Part model, mm, in its own coordinate system. Face numbers are marked on the shaded views. A direction names the side the tool comes from. Coordinates: 2 decimals unless noted, no trailing zeros. Write each loop counter-clockwise with the first axis right and the second up, starting at its lowest first coordinate (ties: lowest second). Pieces come first, ordered by that corner, then holes. Notation, with made-up numbers: M -12,17 L 41,17 A14 ccw 41,32 Z; hole C 11,3.5 d8. An arc over 180 degrees is marked long. Use a Markdown table: item, result. Add a question column.
Q1. Mould opens along X. For the marked faces 5, 6 and 7 say: released by +X, released by -X, zero draft, split by the parting line, or undercut.
Q2. Slice it at D-D on y = 100. Write the cut outline in (x, z).
Q3. Pin check, flat tips, straight feed: pin 1 Ø8 at (x, z) = (170, 58) entering from +Y; pin 2 Ø6 at (x, z) = (7.5, 183) entering from +Y. Stop position of each tip, or through.
Q4. Slice it at B-B on z = 300. Write the cut outline in (x, y), then the cut area to 3 significant figures.
Q5. Tool access for the marked faces 1, 2, 3 and 4: list every direction of +Z, -Z, +X, -X, +Y, -Y with a clear straight run to the whole face (end or side of a thin tool).
Q6. Slice it at C-C on x = 202.5. Write the cut outline in (y, z), then the cut area to 3 significant figures.
Q7. Slice it at A-A on y = 179. Write the cut outline in (x, z).
Q8. Wall check: L1, parallel to X at y = 167.5, z = 113; L2, parallel to Z at x = -142, y = 162.5; L3, parallel to X at y = 118.5, z = 130. Give the ranges that are in metal, low to high. Write a range as from..to.
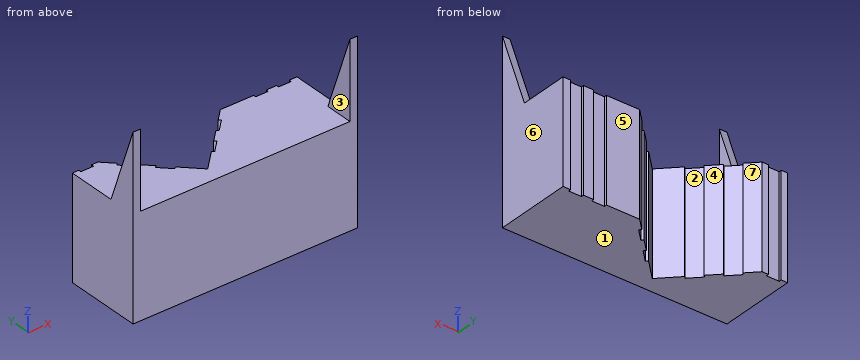
Autodesk Inventor part; units mm, degrees
ref_plane "YZ Plane" through (0, 0, 0) normal (1, 0, 0) x (0, 1, 0)
ref_plane "XZ Plane" through (0, 0, 0) normal (0, 1, 0) x (-1, 0, 0)
ref_plane "XY Plane" through (0, 0, 0) normal (0, 0, 1) x (1, 0, 0)
sketch "Sketch1" plane through (0, 0, 0) normal (0, 0, 1) x (1, 0, 0)
  line L0 (-190.0993, 60.6039) -> (-190.0993, 210.6039)
  line L1 (149.9007, 210.6039) -> (149.9007, 60.6039)
  line L2 (149.9007, 60.6039) -> (-190.0993, 60.6039)
  line L3 (149.9007, 210.6039) -> (249.9007, 210.6039)
  line L4 (249.9007, 210.6039) -> (249.9007, 60.6039)
  line L5 (249.9007, 60.6039) -> (149.9007, 60.6039)
  line L6 (-190.0993, 210.6039) -> (-140.0993, 210.6039)
  line L7 (-140.0993, 210.6039) -> (-20.0993, 90.6039)
  line L8 (-20.0993, 90.6039) -> (99.9007, 210.6039)
  line L9 (99.9007, 210.6039) -> (149.9007, 210.6039)
  point P0 (0, 0)
  dimension "d0" = 340
  dimension "d1" = 150
  dimension "d2" = 150
  dimension "d3" = 170
  dimension "d5" = 100
  dimension "d16" = 90
  dimension "d17" = 50
  dimension "d18" = 50
extrude "Extrusion1" add sketch "Sketch1" along normal blind 200
sketch "Sketch2" plane through (0, 0, 200) normal (0, 0, 1) x (1, 0, 0)
  point P0 (0, 0)
sketch "Sketch3" plane through (249.9007, 60.6039, 0) normal (1, 0, 0) x (0, 0, -1)
  line L0 (0, 0) -> (0, 150)
  line L1 (0, 150) -> (-200, 150)
  line L2 (-200, 0) -> (-200, 150)
  line L3 (0, 0) -> (-200, 0)
  line L4 (-200, 0) -> (-350, 0)
  line L5 (-350, 0) -> (-200, 54.5955)
  line L6 (-200, 0) -> (-200, 150)
  point P0 (0, -60.6039)
  dimension "d12" = 20
  dimension "d13" = 150
extrude "Extrusion2" add sketch "Sketch3" against normal blind 15 contours L4 L5 L2
sketch "Sketch4" plane through (-190.0993, 60.6039, 0) normal (-1, 0, 0) x (0, 0, 1)
  line L0 (200, 0) -> (200, 54.5955)
  line L1 (200, 0) -> (350, 0)
  line L2 (350, 0) -> (200, 54.5955)
  point P0 (0, -60.6039)
extrude "Extrusion3" add sketch "Sketch4" against normal blind 15
sketch "Sketch5" plane through (0, 0, 200) normal (0, 0, 1) x (1, 0, 0)
  line L0 (-119.0942, 189.5988) -> (-122.6298, 186.0633)
  line L1 (-122.6298, 186.0633) -> (-101.4166, 164.8501)
  line L2 (-101.4166, 164.8501) -> (-97.881, 168.3856)
  line L3 (-20.0993, 90.6039) -> (-140.0993, 210.6039)
  line L4 (-76.6678, 147.1724) -> (-80.2034, 143.6369)
  line L5 (-80.2034, 143.6369) -> (-58.9902, 122.4237)
  line L6 (-58.9902, 122.4237) -> (-55.4546, 125.9592)
  line L7 (-20.0993, 90.6039) -> (-20.0993, 149.2833) construction
  line L8 (78.8957, 189.5988) -> (82.4312, 186.0633)
  line L9 (82.4312, 186.0633) -> (61.218, 164.8501)
  line L10 (61.218, 164.8501) -> (57.6825, 168.3856)
  line L11 (36.4693, 147.1724) -> (40.0048, 143.6369)
  line L12 (40.0048, 143.6369) -> (18.7916, 122.4237)
  line L13 (18.7916, 122.4237) -> (15.256, 125.9592)
  line L14 (-175.0993, 115.1994) -> (-175.0993, 60.6039)
  line L15 (-175.0993, 60.6039) -> (234.9007, 60.6039)
  line L16 (234.9007, 60.6039) -> (234.9007, 115.1994)
  line L17 (234.9007, 115.1994) -> (249.9007, 115.1994)
  line L18 (249.9007, 115.1994) -> (249.9007, 210.6039)
  line L19 (249.9007, 210.6039) -> (99.9007, 210.6039)
  line L20 (99.9007, 210.6039) -> (-20.0993, 90.6039)
  line L21 (-20.0993, 90.6039) -> (-140.0993, 210.6039)
  line L22 (-140.0993, 210.6039) -> (-190.0993, 210.6039)
  line L23 (-190.0993, 210.6039) -> (-190.0993, 115.1994)
  line L24 (-190.0993, 115.1994) -> (-175.0993, 115.1994)
  line L25 (249.9007, 210.6039) -> (99.9007, 210.6039)
  line L26 (164.9007, 210.6039) -> (164.9007, 205.6039)
  line L27 (164.9007, 205.6039) -> (189.9007, 205.6039)
  line L28 (189.9007, 205.6039) -> (189.9007, 210.6039)
  line L29 (209.9007, 210.6039) -> (209.9007, 205.6039)
  line L30 (209.9007, 205.6039) -> (234.9007, 205.6039)
  line L31 (234.9007, 205.6039) -> (234.9007, 210.6039)
  line L32 (-140.0993, 210.6039) -> (-190.0993, 210.6039)
  line L33 (-177.5993, 210.6039) -> (-177.5993, 205.6039)
  line L34 (-177.5993, 205.6039) -> (-152.5993, 205.6039)
  line L35 (-152.5993, 205.6039) -> (-152.5993, 210.6039)
  point P0 (0, 0)
  point P1 (78.8957, 189.5988)
  point P2 (57.6825, 168.3856)
  point P3 (36.4693, 147.1724)
  dimension "d19" = 5
  dimension "d20" = 30
  dimension "d21" = 5
  dimension "d22" = 30
  dimension "d23" = 50
  dimension "d24" = 30
  dimension "d27" = 5
  dimension "d28" = 25
  dimension "d29" = 25
  dimension "d30" = 20
  dimension "d31" = 15
  dimension "d32" = 25
  dimension "d33" = 12.5
  dimension "d34" = 5
extrude "Extrusion4" cut sketch "Sketch5" against normal up to surface (200 mm away) contours L3 L2 L1 L0 | L3 L6 L5 L4 | L35 L34 L33 L22 | L20 L11 L12 L13 | L20 L8 L9 L10 | L19 L28 L27 L26 | L19 L31 L30 L29
equation "\"d2\" = d1"
equation "\"d3\" = 0.5 * d0"
equation "\"d18\" = d17"
equation "\"d21\" = d19"
equation "\"d22\" = d20"
equation "\"d27\" = d19"
equation "\"d29\" = d28"
properties part number "Modelo base"
Recorded:
| question | item | result |
|---|---|---|
| 1 | face 5 | zero draft |
| 1 | face 6 | released by +X |
| 1 | face 7 | undercut |
| 2 | outline | M -190.1,0 L -29.5,0 L -29.5,200 L -175.1,200 L -175.1,241.76 L -190.1,241.76 Z; M -10.7,0 L 249.9,0 L 249.9,241.76 L 234.9,241.76 L 234.9,200 L -10.7,200 Z |
| 3 | pin 1 | y = 205.6 |
| 3 | pin 2 | y = 121.2 |
| 4 | outline | M -190.1,60.6 L -175.1,60.6 L -175.1,78.8 L -190.1,78.8 Z; M 234.9,60.6 L 249.9,60.6 L 249.9,78.8 L 234.9,78.8 Z |
| 4 | area | 546 mm² |
| 5 | face 1 | -Z, +X, -X, +Y, -Y |
| 5 | face 2 | +Z, -Z |
| 5 | face 3 | +Z, +Y, -Y |
| 5 | face 4 | +Z, -Z, +Y |
| 6 | outline | M 60.6,0 L 210.6,0 L 210.6,200 L 60.6,200 Z |
| 6 | area | 30,000 mm² |
| 7 | outline | M -190.1,0 L -115.57,0 L -115.57,200 L -190.1,200 Z; M 75.37,0 L 249.9,0 L 249.9,200 L 75.37,200 Z |
| 8 | L1 | -190.1..-104.07, -98.77..-97, 56.8..58.57, 63.87..249.9 |
| 8 | L2 | 0..200 |
| 8 | L3 | -190.1..-48, 7.8..249.9 |
